```python
from build123d import *

# Parameters (mm, degrees)
F0_W     = 381
F0_H     = 381
F0_R     = 6.35
F0_W_2   = 330.2
F0_H_2   = 330.2
F1_DEPTH = 6.35
F0_W_3   = 317.5
F0_H_3   = 317.5
F2_DEPTH = 50.8


with BuildPart() as f1:
    # F0 (on Top) → F1 (new body)
    with BuildSketch(Plane.XY):
        with Locations((15.531801, -4.447729)):
            Rectangle(F0_W, F0_H)
        with Locations((-162.268199, -182.247729)):
            Circle(F0_R, mode=Mode.SUBTRACT)
        with Locations((193.331801, -182.247729)):
            Circle(F0_R, mode=Mode.SUBTRACT)
        with Locations((-162.268199, 173.352271)):
            Circle(F0_R, mode=Mode.SUBTRACT)
        with Locations((15.531801, -4.447729)):
            Rectangle(F0_W_2, F0_H_2, mode=Mode.SUBTRACT)
        with Locations((193.331801, 173.352271)):
            Circle(F0_R, mode=Mode.SUBTRACT)
    extrude(amount=F1_DEPTH)

    # F0 (on Top) → F2 (join)
    with BuildSketch(Plane.XY):
        with Locations((15.531801, -4.447729)):
            Rectangle(F0_W_2, F0_H_2)
        with Locations((15.531801, -4.447729)):
            Rectangle(F0_W_3, F0_H_3, mode=Mode.SUBTRACT)
    extrude(amount=F2_DEPTH)


solid = f1.part
```
Geometry: final body of the model. Coordinates: model frame, mm. A direction names the side the tool comes from. Coordinates: 2 decimals unless noted, no trailing zeros. Order: outer loops, then holes, each group sorted by start corner. A loop starts at its lowest first (then second) coordinate and runs counter-clockwise, first axis right, second up. Notation, with made-up numbers: M -34,-38 L -7,-38 A21 cw -7,-33 Z; hole C 31,66.25 d5. An arc over 180 degrees is marked long. Answer as CSV lines item,"result".
Q1. Set-up query: faces 1 (the flat face through (13, -169.548, 28)), 2 (the flat face through (-144, 70, 50.8)), 3 (the flat face through (-149.568, -7, 28)), 4 (the flat face through (13, 154.302, 25)). Return all of +Z, -Z, +X, -X, +Y, -Y with unobstructed straight access to the full face (end or side cutting, diameter ignored); none if empty.
Answers:
face 1,"+Z, +X, -X, -Y"
face 2,"+Z, +X, -X, +Y, -Y"
face 3,"+Z, -X, +Y, -Y"
face 4,"+Z, -Z"
Q2. Section C-C on x = 138.5. Return the cut outline in (y, z), and give its area (3 significant figures).
Answers:
outline,"M -194.95,0 L -163.2,0 L -163.2,50.8 L -169.55,50.8 L -169.55,6.35 L -194.95,6.35 Z; M 154.3,0 L 186.05,0 L 186.05,6.35 L 160.65,6.35 L 160.65,50.8 L 154.3,50.8 Z"
area,"968 mm^2"
Q3. Draft query along Y for faces 5 (the cylindrical face through (-159.338, -187.881, 3.131)), 6 (the flat face through (180.632, -7, 28)), 7 (the flat face through (13, 160.652, 28)). Return one class per face: pulls with the +Y half, pulls with the -Y half, needs draft (parallel to the pull), parting line crosses it, or undercut.
Answers:
face 5,"undercut"
face 6,"needs draft"
face 7,"pulls with the +Y half"
Q4. Section A-A on z = 14.5. Return the cut outline in (x, y).
Answers:
outline,"M -149.57,-169.55 L 180.63,-169.55 L 180.63,160.65 L -149.57,160.65 Z; hole M -143.22,-163.2 L 174.28,-163.2 L 174.28,154.3 L -143.22,154.3 Z"
Q5. First-contact query: P1, Ø4, axis at x = 72.5, z = 41, coming from the -Y side; P2, Ø6, axis at x = 146.5, z = 7, coming from the +Y side; P3, Ø8, axis at y = 142.5, z = 40.5, coming from the -X side; P4, Ø20.5, axis at x = -162.27, y = 173.35, coming from the +Z side. Flat tips, straight axial feed; report the tip coordinate or a pass-through.
Answers:
P1,"stops at y = -169.55"
P2,"stops at y = 186.05"
P3,"stops at x = -149.57"
P4,"stops at z = 6.35"
Q6. Section B-B on y = -127. Return the cut outline in (x, z).
Answers:
outline,"M -174.97,0 L -143.22,0 L -143.22,50.8 L -149.57,50.8 L -149.57,6.35 L -174.97,6.35 Z; M 174.28,0 L 206.03,0 L 206.03,6.35 L 180.63,6.35 L 180.63,50.8 L 174.28,50.8 Z"
Q7. Line query: probe 1 along Y at (x, z) = (107, 7.5); probe 2 along X at (y, z) = (91, 13.5); probe 3 along Y at (x, z) = (143, 6). Output: solid intervals per line, ascending. Write a range as [from, to].
Answers:
probe 1,"y = [-169.55, -163.2], [154.3, 160.65]"
probe 2,"x = [-149.57, -143.22], [174.28, 180.63]"
probe 3,"y = [-194.95, -163.2], [154.3, 186.05]"
